Check sheet for the modelled part. Datum: model origin and axes. Units: mm. Give positions to 0.01 mm unless a question says otherwise; leave off trailing zeros. Write each loop counter-clockwise with the first axis right and the second up, starting at its lowest first coordinate (ties: lowest second). Pieces come first, ordered by that corner, then holes. Notation, with made-up numbers: (-30, 32.5) -> (14, 32.5) arc R30 cw to (14, 68.5) -> close; hole circle Ø10 at (61.5, 40.5). An arc over 180 degrees is marked (long way). Answer as a JSON object with one key per item and string values.
from build123d import *

# Parameters (mm, degrees)
SKETCH1_R           = 2.0701
BOSS_EXTRUDE1_DEPTH = 2.286


with BuildPart() as part:
    # Sketch1 → Boss-Extrude1 (new body)
    with BuildSketch(Plane(origin=(0, 0, 0), x_dir=(-1, 0, 0), z_dir=(0, 0, -1))):
        with BuildLine():
            Line((-29.230637652, -76.282949552), (-16.965734073, -55.039513402))
            ThreePointArc((-16.965734073, -55.039513402), (-14.394339663, -53.974406963), (-12.7, -56.182513402))
            Line((-12.7, -56.182513402), (-12.7, -80.682217477))
            Line((-12.7, -80.682217477), (-11.617101368, -82.55))
            Line((-11.617101368, -82.55), (10.832217477, -82.55))
            Line((10.832217477, -82.55), (12.7, -81.467101368))
            Line((12.7, -81.467101368), (12.7, 8.779535349))
            Line((12.7, 8.779535349), (11.617101368, 10.647317872))
            Line((11.617101368, 10.647317872), (-4.632676327, 14.969773631))
            Line((-4.632676327, 14.969773631), (-6.50045885, 13.886874999))
            Line((-6.50045885, 13.886874999), (-51.625488503, -64.271969053))
            Line((-51.625488503, -64.271969053), (-50.542589871, -66.139751576))
            Line((-50.542589871, -66.139751576), (-31.098420176, -77.365848184))
            Line((-31.098420176, -77.365848184), (-29.230637652, -76.282949552))
        make_face()
        with Locations((-38.1, -65.991135768)):
            Circle(SKETCH1_R, mode=Mode.SUBTRACT)
        with Locations((0, -63.5)):
            Circle(SKETCH1_R, mode=Mode.SUBTRACT)
        with Locations((-25.4, -43.994090512)):
            Circle(SKETCH1_R, mode=Mode.SUBTRACT)
        with Locations((-12.7, -21.997045256)):
            Circle(SKETCH1_R, mode=Mode.SUBTRACT)
        with Locations((0, -38.1)):
            Circle(SKETCH1_R, mode=Mode.SUBTRACT)
        with Locations((0, -12.7)):
            Circle(SKETCH1_R, mode=Mode.SUBTRACT)
        Circle(SKETCH1_R, mode=Mode.SUBTRACT)
        with Locations((-6.35, -10.998522628)):
            Circle(SKETCH1_R, mode=Mode.SUBTRACT)
        with Locations((0, -25.4)):
            Circle(SKETCH1_R, mode=Mode.SUBTRACT)
        with Locations((0, -50.8)):
            Circle(SKETCH1_R, mode=Mode.SUBTRACT)
        with Locations((-19.05, -32.995567884)):
            Circle(SKETCH1_R, mode=Mode.SUBTRACT)
        with Locations((-31.75, -54.99261314)):
            Circle(SKETCH1_R, mode=Mode.SUBTRACT)
        with Locations((0, -76.2)):
            Circle(SKETCH1_R, mode=Mode.SUBTRACT)
    extrude(amount=-BOSS_EXTRUDE1_DEPTH)


solid = part.part
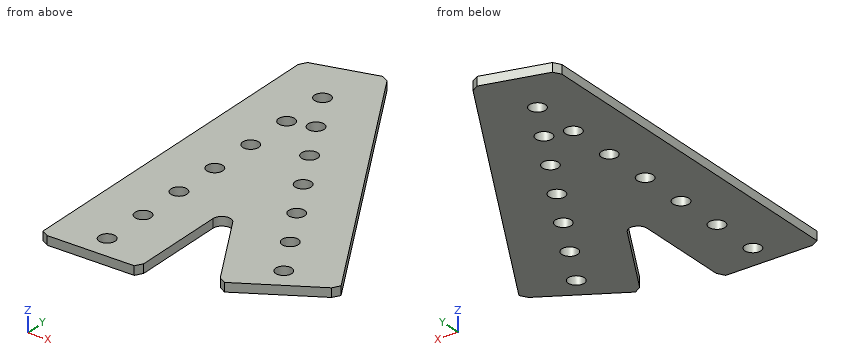
1. Sectioned sample at A-A, the plane x = 38.1. Enter the section's corners in (y, z), plus the area to 3 significant figures.
Determined:
{"outline": "(-73.32, 0) -> (-68.06, 0) -> (-68.06, 2.29) -> (-73.32, 2.29) -> close; (-63.92, 0) -> (-40.85, 0) -> (-40.85, 2.29) -> (-63.92, 2.29) -> close", "area": "64.8 mm^2"}
2. Sectioned sample at D-D, the plane x = 25. Enter the section's corners in (y, z), plus the area to 3 significant figures.
Determined:
{"outline": "(-68.96, 0) -> (-46.03, 0) -> (-46.03, 2.29) -> (-68.96, 2.29) -> close; (-41.96, 0) -> (-18.16, 0) -> (-18.16, 2.29) -> (-41.96, 2.29) -> close", "area": "107 mm^2"}
3. Scan lines: L1, parallel to Y at x = 6.35, z = 0.6; L2, parallel to Y at x = 32, z = 0.95; L3, parallel to X at y = -22, z = 0.2. Record each from-to range of solid material in increasing order. Write a range as [from, to].
Determined:
{"L1": "[-82.55, -13.07], [-8.93, 13.97]", "L2": "[-76.85, -57.05], [-52.94, -30.28]", "L3": "[-12.7, 10.63], [14.77, 27.22]"}
4. Sectioned sample at B-B, the plane z = 0.9. State how many separate pieces and enclosed holes the cut face has, plus the area to 3 significant figures.
Determined:
{"separate pieces": "1", "enclosed holes": "13", "area": "3,670 mm^2"}
